Could you check a few things on this model? Use its own coordinates, in mm. Face numbers are marked on the shaded views. A direction names the side the tool comes from. Round coordinates to 2 decimals unless told otherwise and drop trailing zeros. Loops run counter-clockwise (first coordinate to the right, second up) from the corner with the lowest first, then second, coordinate; pieces in that order, holes last.
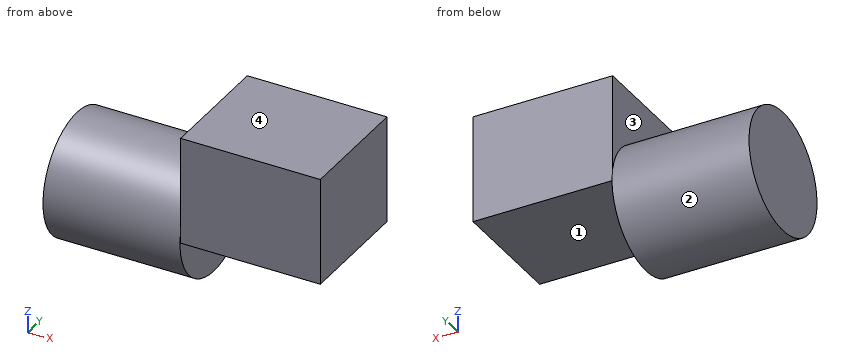
from build123d import *

# Parameters (mm, degrees)
F1_DEPTH = 25
F0_W     = 57.5316473842
F0_H     = 25.4905093461


with BuildPart() as f1:
    # F0 (on Front) → F1 (new body, symmetric)
    with BuildSketch(Plane.XZ):
        Polygon((0, 25.4905093461), (0, 0), (58.6708895862, 0), (58.6708895862, 45.1424047351), (0, 45.1424047351), align=None)
    extrude(amount=F1_DEPTH, both=True)

    # F0 (on Front) → F2 (revolve)
    with BuildSketch(Plane.XZ):
        with Locations((-28.7658236921, 12.7452546731)):
            Rectangle(F0_W, F0_H)
    revolve(axis=Axis((-28.7658236921, 0, 0), (-1, 0, 0)))


solid = f1.part
Item 1: If we section it at D-D, the plane x = 12: Please give me the cut outline in (y, z).
Results list:
outline: (-25, 0) - (25, 0) - (25, 45.14) - (-25, 45.14) - close
Item 2: For the marked faces 1, 2, 3 and 4, which set-ups out of +Z, -Z, +X, -X, +Y, -Y let a thin tool reach every point of the face, with its end or its side?
Results list:
face 1: -Z, +X, +Y, -Y
face 2: -X
face 3: +Z, -X
face 4: +Z, +X, -X, +Y, -Y
Item 3: If we section it at A-A, the plane y = 0: Please give me the cut outline in (x, z).
Results list:
outline: (-57.53, -25.49) - (0, -25.49) - (0, 0) - (58.67, 0) - (58.67, 45.14) - (0, 45.14) - (0, 25.49) - (-57.53, 25.49) - close
Item 4: If we section it at B-B, the plane z = 17: Please give me the cut outline in (x, y).
Results list:
outline: (-57.53, -18.99) - (0, -18.99) - (0, -25) - (58.67, -25) - (58.67, 25) - (0, 25) - (0, 18.99) - (-57.53, 18.99) - close
Item 5: If I drill on line 1 along X through (y, z) = (-17, -9); line 2 along Y through (x, z) = (35, 32.5); line 3 along Z through (x, y) = (38, 16), over which ranges is the centre line in solid material (lowest first)?
Results list:
line 1: x = -57.53 to 0
line 2: y = -25 to 25
line 3: z = 0 to 45.14
Item 6: If we section it at C-C, the plane x = -13: Please give me the cut outline in (y, z).
Results list:
outline: circle Ø50.98 at (0, 0)
Item 7: Will these pins go through, and if not, where does the flat tip stop? pin 1 (8 mm diameter, centred on x = -11.5, z = -11, fed in from -Y); pin 2 (13.5 mm diameter, centred on x = 40, z = 13.5, fed in from +Y); pin 3 (1 mm diameter, centred on x = -14.5, y = 4, fed in from -Z).
Results list:
pin 1: stops at y = -24.51
pin 2: stops at y = 25
pin 3: stops at z = -25.25
